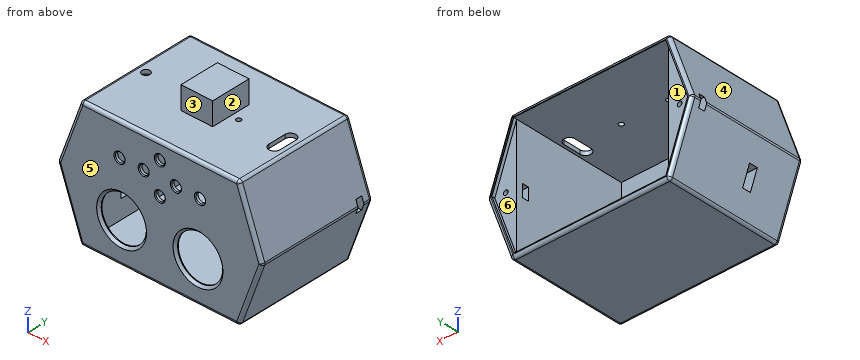
Autodesk Inventor part; units mm, degrees
ref_plane "YZ Plane" through (0, 0, 0) normal (1, 0, 0) x (0, 1, 0)
ref_plane "XZ Plane" through (0, 0, 0) normal (0, 1, 0) x (-1, 0, 0)
ref_plane "XY Plane" through (0, 0, 0) normal (0, 0, 1) x (1, 0, 0)
sketch "Sketch4" plane through (0, 0, 0) normal (0, 1, 0) x (-1, 0, 0)
  line L0 (50, 40.5) -> (-50, 40.5)
  line L1 (-50, 40.5) -> (-50, -40.5)
  line L2 (-50, -40.5) -> (50, -40.5)
  line L3 (50, -40.5) -> (50, 40.5)
  line L4 (50, 40.5) -> (-50, -40.5) construction
  line L5 (-50, 40.5) -> (50, -40.5) construction
  line L6 (45.72, 36.195) -> (-45.72, 36.195)
  line L7 (-45.72, 36.195) -> (-45.72, -36.195)
  line L8 (-45.72, -36.195) -> (45.72, -36.195)
  line L9 (45.72, -36.195) -> (45.72, 36.195)
  line L10 (45.72, 36.195) -> (-45.72, -36.195) construction
  line L11 (-45.72, 36.195) -> (45.72, -36.195) construction
  line L12 (48, 38) -> (-48, 38)
  line L13 (-48, 38) -> (-48, -38)
  line L14 (-48, -38) -> (48, -38)
  line L15 (48, -38) -> (48, 38)
  line L16 (48, 38) -> (-48, -38) construction
  line L17 (-48, 38) -> (48, -38) construction
  line L18 (-50, 40.5) -> (-64.7408, 0)
  line L19 (-50, 40.5) -> (-6.9008, 40.5) construction
  line L20 (-50, -40.5) -> (-64.7408, 0)
  line L21 (-50, -40.5) -> (-6.9008, -40.5) construction
  line L22 (0, 0) -> (72.39, 0) construction
  line L23 (0, -40.5) -> (0, 40.5)
  line L24 (50, 40.5) -> (64.7408, 0)
  line L25 (50, -40.5) -> (64.7408, 0)
  line L26 (64.7408, 0) -> (-64.7408, 0)
  circle A0 centre (25.4, 19.685) radius 3
  circle A1 centre (10.16, 19.685) radius 3
  circle A2 centre (-25.4, 19.685) radius 3
  circle A3 centre (-10.16, 19.685) radius 3
  circle A4 centre (0, 29.845) radius 3
  circle A5 centre (0, 9.525) radius 3
  line L27 (45.72, -36.195) -> (48.26, -36.195) construction
  line L28 (43.18, -33.655) -> (5.08, -33.655)
  line L29 (5.08, -33.655) -> (5.08, 4.445)
  line L30 (5.08, 4.445) -> (43.18, 4.445)
  line L31 (43.18, 4.445) -> (43.18, -33.655)
  line L32 (5.08, -14.605) -> (24.13, -14.605) construction
  circle A6 centre (24.13, -14.605) radius 14.25
  line L33 (-43.18, -33.655) -> (-5.08, -33.655)
  line L34 (-5.08, -33.655) -> (-5.08, 4.445)
  line L35 (-5.08, 4.445) -> (-43.18, 4.445)
  line L36 (-43.18, 4.445) -> (-43.18, -33.655)
  circle A7 centre (-24.13, -14.605) radius 14.25
  line L37 (-48, -38) -> (-61.8309, 0)
  line L38 (-48, -38) -> (-7.5612, -38) construction
  line L39 (-48, 38) -> (-61.8309, 0)
  line L40 (-48, 38) -> (-7.5612, 38) construction
  line L41 (48, -38) -> (61.8309, 0)
  line L42 (48, 38) -> (61.8309, 0)
  circle A8 centre (54.9155, 0) radius 1.5
  circle A9 centre (-54.9155, 0) radius 1.5
  point P0 (0, 36.195)
  dimension "d52" = 100
  dimension "d53" = 81
  dimension "d54" = 91.44
  dimension "d55" = 72.39
  dimension "d56" = 96
  dimension "d57" = 76
  dimension "d58" = 110
  dimension "d59" = 110
  dimension "d62" = 6
  dimension "d63" = 20.32
  dimension "d64" = 16.51
  dimension "d65" = 6
  dimension "d66" = 15.24
  dimension "d67" = 6
  dimension "d68" = 6.35
  dimension "d69" = 6
  dimension "d70" = 20.32
  dimension "d73" = 38.1
  dimension "d74" = 38.1
  dimension "d75" = 2.54
  dimension "d76" = 2.54
  dimension "d79" = 28.5
  dimension "d83" = 110
  dimension "d84" = 110
  dimension "d86" = 3
  dimension "d112" = 54.9155
extrude "Extrusion7" add sketch "Sketch4" along normal blind 76 contours L3 L42 L12 L23 L0 | L24 L26 L42 L3 | L23 L12 L39 L1 L0 | L25 L3 L41 L26 | L1 L39 L26 L18 | L2 L23 L14 L41 L3 | L26 L37 L1 L20 | L2 L1 L37 L14 L23
extrude "Extrusion8" add sketch "Sketch4" along normal blind 74 contours L42 L26 A8 L3 | L3 L26 L15 L42 | L26 A8 L41 L3 | L3 L41 L15 L26 | L39 L13 L26 L1 | L1 L26 A9 L39 | L26 L13 L37 L1 | L1 L37 L26 A9
fillet "Fillet4" radius 2 18 edges at (0, 0, -40.5) (-50, 38, -40.5) (0, 76, -40.5) (50, 38, -40.5) (57.3704, 0, -20.25) (57.3704, 76, -20.25) (64.7408, 38, 0) (57.3704, 0, 20.25) (57.3704, 76, 20.25) (50, 38, 40.5) (-57.3704, 0, 20.25) (-50, 38, 40.5) (-57.3704, 76, 20.25) (-64.7408, 38, 0) (0, 0, 40.5) (-57.3704, 0, -20.25) (0, 76, 40.5) (-57.3704, 76, -20.25)
extrude "Extrusion11" add sketch "Sketch4" along normal blind 70 contours A8 L26 | L26 A8 | A9 L26 | L26 A9
sketch "Sketch5" plane through (-48.5996, 74, 40.5) normal (0, 0, 1) x (1, 0, 0)
  line L0 (0, -72) -> (97.1992, -72)
  line L1 (97.1992, -72) -> (0, -72)
  line L2 (97.1992, 0) -> (0, 0)
  line L3 (0, -72) -> (0, 0)
  line L4 (0, 0) -> (97.1992, 0)
  line L5 (97.1992, 0) -> (97.1992, -72)
  line L6 (97.1992, -36) -> (0, -36)
  line L7 (48.5996, -72) -> (48.5996, 0)
  line L8 (58.5996, -23.5) -> (38.5996, -23.5)
  line L9 (38.5996, -23.5) -> (38.5996, -48.5)
  line L10 (38.5996, -48.5) -> (58.5996, -48.5)
  line L11 (58.5996, -48.5) -> (58.5996, -23.5)
  line L12 (58.5996, -23.5) -> (38.5996, -48.5) construction
  line L13 (38.5996, -23.5) -> (58.5996, -48.5) construction
  circle A0 centre (33.5996, -36) radius 1.5
  circle A1 centre (63.5996, -36) radius 1.5
  line L14 (67.8423, -21) -> (29.3569, -21)
  line L15 (29.3569, -21) -> (29.3569, -51)
  line L16 (29.3569, -51) -> (67.8423, -51)
  line L17 (67.8423, -51) -> (67.8423, -21)
  line L18 (67.8423, -21) -> (29.3569, -51) construction
  line L19 (29.3569, -21) -> (67.8423, -51) construction
  line L20 (91.1992, -30.5) -> (91.1992, -41.5) construction
  line L21 (87.6992, -30.5) -> (87.6992, -41.5)
  line L22 (94.6992, -41.5) -> (94.6992, -30.5)
  arc A2 (94.6992, -30.5) -> (87.6992, -30.5) centre (91.1992, -30.5) ccw
  arc A3 (87.6992, -41.5) -> (94.6992, -41.5) centre (91.1992, -41.5) ccw
  line L23 (97.1992, 0) -> (97.1992, -72)
  circle A4 centre (5, -36) radius 2.5
  line L24 (0, -72) -> (0, 0)
  point P0 (48.5996, -74)
  point P1 (48.5996, -36)
  point P2 (91.1992, -36)
  dimension "d115" = 20
  dimension "d118" = 3
  dimension "d119" = 15
  dimension "d134" = 25
  dimension "d135" = 30
  dimension "d176" = 5.5
  dimension "d177" = 7
  dimension "d178" = 6
  dimension "d179" = 5
  dimension "d180" = 5
extrude "Extrusion12" add sketch "Sketch5" along normal blind 14.5 contours L10 L9 L6 L7 | L7 L6 L11 L10 | L7 L8 L11 L6 | L6 L9 L8 L7
extrude "Extrusion14" cut sketch "Sketch5" along normal blind 10 and the other way blind 5 contours A0 L6 | L6 A0 | A1 L6 | L6 A1
extrude "Extrusion15" add sketch "Sketch4" along normal blind 2 contours L23 L6 L7 L26 L13 L12 | L12 L15 L26 L9 L6 L23 | L23 A4 A5 L26 L34 L35 L36 L7 L6 | L6 L9 L26 L31 L30 L29 L23 A5 A4 | L15 L14 L23 L8 L9 L26 | L26 L7 L8 L23 L14 L13 | L9 L8 L23 L26 L29 L28 L31 | L26 L36 L33 L34 L23 L8 L7 | L31 L28 L29 L26 | L26 L29 L30 L31 | L36 L35 L34 L26 | L26 L34 L33 L36
chamfer "Chamfer10" distance 1.5 angle 45 2 edges at (38.38, 0, -14.605) (-9.88, 0, -14.605)
chamfer "Chamfer11" distance 0.5 angle 45 6 edges at (28.4, 0, 19.685) (13.16, 0, 19.685) (3, 0, 9.525) (-7.16, 0, 19.685) (3, 0, 29.845) (-22.4, 0, 19.685)
extrude "Extrusion16" cut sketch "Sketch5" against normal up to surface (2.5 mm away) contours A4 L6 | L6 A4 | L22 A3 L21 L6 | L6 L21 A2 L22
sketch "Sketch6" plane through (-48, 74, 38) normal (1, 0, 0) x (0, 0, -1)
  line L0 (38, -4) -> (42, -4)
  line L1 (42, -4) -> (42, -8)
  line L2 (42, -8) -> (38, -8)
  line L3 (38, -8) -> (38, -4)
  line L4 (38, -4) -> (38, -8)
  line L5 (38, -8) -> (34, -8)
  line L6 (34, -8) -> (34, -4)
  line L7 (34, -4) -> (38, -4)
  line L8 (0, 0) -> (76, 0)
  point P0 (38, -74)
  point P1 (38, 0)
  dimension "d183" = 4
  dimension "d184" = 4
  dimension "d185" = 4
  dimension "d186" = 4
extrude "Extrusion17" cut sketch "Sketch6" along normal through all both and the other way through all
sketch "Sketch7" plane through (0, 0, 0) normal (1, 0, 0) x (0, 1, 0)
  line L0 (0, 0) -> (0, 38.5)
  line L1 (74, 0) -> (76, 0)
  line L2 (0, 0) -> (76, 0)
  line L3 (0, 0) -> (76, 0)
  line L4 (76, 0) -> (76, -40.5)
  line L5 (76, -40.5) -> (0, -40.5)
  line L6 (0, -40.5) -> (0, 0)
  line L7 (76, 0) -> (76, 40.5)
  line L8 (76, 40.5) -> (0, 40.5)
  line L9 (0, 40.5) -> (0, 0)
  line L10 (31, 0) -> (31, -40.5)
  line L11 (25.5148, 0) -> (25.8682, -40.5)
  line L12 (25.6369, -14) -> (31, -14)
  line L13 (25.7417, -26) -> (31.062, -26)
  point P0 (31, -26)
  dimension "d189" = 40.5
  dimension "d190" = 45
  dimension "d191" = 0.5
  dimension "d192" = 14
  dimension "d193" = 12
extrude "Extrusion18" cut sketch "Sketch7" against normal through all contours L12 L10 L13 L11
properties part number "ControllerHead"
Input: part model. Units: mm. Frame: model coordinates. Face numbers are marked on the shaded views. A direction names the side the tool comes from. Round coordinates to 2 decimals unless told otherwise and drop trailing zeros. Order: outer loops, then holes, each group sorted by start corner. A loop starts at its lowest first (then second) coordinate and runs counter-clockwise, first axis right, second up.
1. Pin query (flat end, axial travel): P1, Ø1.5, axis at x = 33, z = 2.5, coming from the +Y side; P2, Ø7, axis at y = 38, z = 48, coming from the -X side; P3, Ø5, axis at y = 33, z = -29.5, coming from the -X side. Return the tip coordinate at first contact, or that it passes through.
The answers:
P1: stops at y = 2
P2: stops at x = -10
P3: stops at x = -54.91
2. Set-up query: the marked faces 1, 2 and 3. Return all of +Z, -Z, +X, -X, +Y, -Y with unobstructed straight access to the full face (end or side cutting, diameter ignored); none if empty.
The answers:
face 1: +Y
face 2: +Z, +X, +Y, -Y
face 3: +Z, +X, -X, -Y
3. Cut plane C-C, the plane x = -44.5. Output: boundary loops of the cut face in (y, z).
The answers:
outline: (0, -38.5) arc R2 ccw to (2, -40.5) - (74, -40.5) arc R2 ccw to (76, -38.5) - (76, -38) - (2, -38) - (2, 38) - (35.67, 38) - (35.67, 40.5) - (2, 40.5) arc R2 ccw to (0, 38.5) - close; (40.33, 38) - (76, 38) - (76, 38.5) arc R2 ccw to (74, 40.5) - (40.33, 40.5) - close
4. Cut plane D-D, the plane y = 42. Output: boundary loops of the cut face in (x, z).
The answers:
outline: (-64.49, -0.68) - (-50.48, -39.18) arc R2 ccw to (-48.6, -40.5) - (48.6, -40.5) arc R2 ccw to (50.48, -39.18) - (64.49, -0.68) arc R2 ccw to (64.49, 0.68) - (50.48, 39.18) arc R2 ccw to (48.6, 40.5) - (46.1, 40.5) - (46.1, 38) - (48, 38) - (48, -38) - (-48, -38) - (-48, 38) - (39.1, 38) - (39.1, 40.5) - (10, 40.5) - (10, 55) - (-10, 55) - (-10, 40.5) - (-48.6, 40.5) arc R2 ccw to (-50.48, 39.18) - (-64.49, 0.68) arc R2 ccw to start
5. Material intervals for line 1 (Y direction, x = -15, z = 38.6); line 2 (Z direction, x = -39, y = 42); line 3 (Z direction, x = -25.4, y = 1.2) (3 decimals), sorted ascending.
The answers:
line 1: y = 0 to 36.5, 39.5 to 76
line 2: z = -40.5 to -38, 38 to 40.5
line 3: z = -40.333 to -29.099, -0.111 to 16.685, 22.685 to 40.333
6. Cut plane B-B, the plane x = 0. Output: boundary loops of the cut face in (y, z) (3 decimals), then the cut area to 3 significant figures.
The answers:
outline: (0, -38.5) arc R2 ccw to (2, -40.5) - (74, -40.5) arc R2 ccw to (76, -38.5) - (76, -38) - (2, -38) - (2, 6.525) - (0.5, 6.525) - (0, 6.025) - close; (0, 13.025) - (0.5, 12.525) - (2, 12.525) - (2, 26.845) - (0.5, 26.845) - (0, 26.345) - close; (0, 33.345) - (0.5, 32.845) - (2, 32.845) - (2, 38) - (76, 38) - (76, 38.5) arc R2 ccw to (74, 40.5) - (50.5, 40.5) - (50.5, 55) - (25.5, 55) - (25.5, 40.5) - (2, 40.5) arc R2 ccw to (0, 38.5) - close
area: 867 mm2
7. Mould query, pull axis X, two halves, no side actions, for the marked faces 4, 5 and 6. Classes: released by +X, released by -X, zero draft, split by the parting line, or undercut.
The answers:
face 4: released by -X
face 5: zero draft
face 6: undercut
8. Cut plane A-A, the plane y = 55. Output: boundary loops of the cut face in (x, z), then the cut area to 3 significant figures.
The answers:
outline: (-64.49, -0.68) - (-50.48, -39.18) arc R2 ccw to (-48.6, -40.5) - (48.6, -40.5) arc R2 ccw to (50.48, -39.18) - (64.49, -0.68) arc R2 ccw to (64.49, 0.68) - (50.48, 39.18) arc R2 ccw to (48.6, 40.5) - (-48.6, 40.5) arc R2 ccw to (-50.48, 39.18) - (-64.49, 0.68) arc R2 ccw to start; hole (-48, -38) - (48, -38) - (48, 38) - (-48, 38) - close
area: 2,000 mm2
